Geometry: final body of the model. Coordinates: model frame, mm. Face numbers are marked on the shaded views. A direction names the side the tool comes from. Round coordinates to 2 decimals unless told otherwise and drop trailing zeros. Loops run counter-clockwise (first coordinate to the right, second up) from the corner with the lowest first, then second, coordinate; pieces in that order, holes last. Notation, with made-up numbers: (-17.5, 50.25) - (-0.5, 50.25) arc R38 cw to (-0.5, 88.25) - close; hole circle Ø6 at (25.5, -12). An arc over 180 degrees is marked (long way). Use CSV: the item, a comma, the result in double quotes.
from build123d import *

# Parameters (mm, degrees)
F1_DEPTH  = 60
F2_R      = 22.25
F3_DEPTH  = 4
F4_R      = 4.25
F5_DEPTH  = 25
F6_R      = 8
F7_DEPTH  = 1
F8_SIZE   = 3.74999
F9_R      = 4.25
F10_DEPTH = 25
F11_R     = 8
F12_DEPTH = 1
F13_SIZE  = 3.74999
F14_R     = 5
F15_R     = 7


# Not quite as in the source:
# - a fillet or chamfer is up to 0.001 mm smaller than in the source, because OpenCascade refuses the exact size


with BuildPart() as f1:
    # F0 (on Right) → F1 (new body)
    with BuildSketch(Plane.YZ):
        Polygon((32.3616418088, -17.0859274204), (32.3616418088, 47.9140725796), (22.3616418088, 47.9140725796), (22.3616418088, -7.0859274204), (-22.6383581912, -7.0859274204), (-22.6383581912, -17.0859274204), align=None)
    extrude(amount=F1_DEPTH)

    # F2 (on face) → F3 (join)
    with BuildSketch(Plane(origin=(0, 0, -17.0859274204), x_dir=(1, 0, 0), z_dir=(0, 0, -1))):
        with Locations((30, -4.8616418088)):
            Circle(F2_R)
    extrude(amount=F3_DEPTH)

    # F4 (on face) → F5 (cut)
    with BuildSketch(Plane(origin=(0, 0, -21.0859274204), x_dir=(1, 0, 0), z_dir=(0, 0, -1))):
        with Locations((30, -4.8616418088)):
            Circle(F4_R)
    extrude(amount=-F5_DEPTH, mode=Mode.SUBTRACT)

    # F6 (on face) → F7 (cut)
    with BuildSketch(Plane.XY.offset(-7.0859274204)):
        with Locations((30, 4.8616418088)):
            Circle(F6_R)
    extrude(amount=-F7_DEPTH, mode=Mode.SUBTRACT)

    # F8 (size 3.75 in the source; OpenCascade refuses exactly that, so slightly less here)
    f8_edges = [f1.edges().sort_by_distance(p)[0] for p in [
        (25.75, 4.861642, -8.085927),
    ]]
    chamfer(f8_edges, length=F8_SIZE)

    # F9 (on face) → F10 (cut)
    with BuildSketch(Plane(origin=(0, 32.3616418088, 0), x_dir=(-1, 0, 0), z_dir=(0, 1, 0))):
        with Locations((-30, 25.9140725796)):
            Circle(F9_R)
    extrude(amount=-F10_DEPTH, mode=Mode.SUBTRACT)

    # F11 (on face) → F12 (cut)
    with BuildSketch(Plane(origin=(0, 32.3616418088, 0), x_dir=(-1, 0, 0), z_dir=(0, 1, 0))):
        with Locations((-30, 25.9140725796)):
            Circle(F11_R)
    extrude(amount=-F12_DEPTH, mode=Mode.SUBTRACT)

    # F13 (size 3.75 in the source; OpenCascade refuses exactly that, so slightly less here)
    f13_edges = [f1.edges().sort_by_distance(p)[0] for p in [
        (34.25, 31.361642, 25.914073),
    ]]
    chamfer(f13_edges, length=F13_SIZE)

    # F14
    f14_edges = [f1.edges().sort_by_distance(p)[0] for p in [
        (0, -22.638358, -12.085927),
        (60, -22.638358, -12.085927),
        (60, 27.361642, 47.914073),
        (0, 27.361642, 47.914073),
    ]]
    fillet(f14_edges, radius=F14_R)

    # F15
    f15_edges = [f1.edges().sort_by_distance(p)[0] for p in [
        (30, 22.361642, -7.085927),
    ]]
    fillet(f15_edges, radius=F15_R)


solid = f1.part
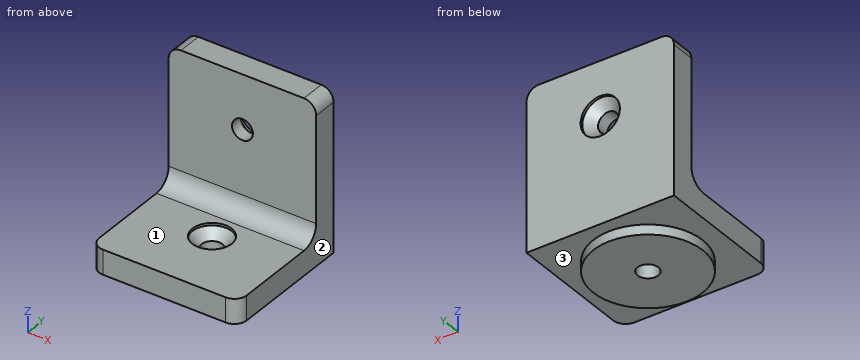
Item 1: Material intervals for line 1 (Z direction, x = 30, y = 32); line 2 (Z direction, x = 30, y = 26.6); line 3 (Y direction, x = 30, z = -18), sorted ascending.
Final values:
line 1,"z = -17.09 to 17.91, 33.91 to 47.91"
line 2,"z = -21.09 to 21.66, 30.16 to 47.91"
line 3,"y = -17.39 to 0.61, 9.11 to 27.11"
Item 2: Section D-D on x = 19.5. Return the cut outline in (y, z) (3 decimals), plus the area to 3 significant figures.
Final values:
outline,"(-22.638, -17.086) - (-14.755, -17.086) - (-14.755, -21.086) - (24.478, -21.086) - (24.478, -17.086) - (32.362, -17.086) - (32.362, 47.914) - (22.362, 47.914) - (22.362, -0.086) arc R7 cw to (15.362, -7.086) - (-22.638, -7.086) - close"
area,"1,270 mm²"
Item 3: Section C-C on z = -13. Return the cut outline in (x, y), plus the area to 3 significant figures.
Final values:
outline,"(0, -17.64) arc R5 ccw to (5, -22.64) - (55, -22.64) arc R5 ccw to (60, -17.64) - (60, 32.36) - (0, 32.36) - close; hole circle Ø8.5 at (30, 4.86)"
area,"3,230 mm²"
Item 4: Pin query (flat end, axial travel): P1, Ø5, axis at x = 30, y = 4.86, coming from the +Z side; P2, Ø10, axis at x = 33, z = 14, coming from the -Y side; P3, Ø8, axis at x = 31, y = 5.5, coming from the +Z side; P4, Ø19, axis at x = 38, y = 2, coming from the +Z side. Return the tip coordinate at first contact, or that it passes through.
Final values:
P1,"passes through"
P2,"stops at y = 22.36"
P3,"stops at z = -10.9"
P4,"stops at z = -7.09"
Item 5: Section B-B on y = -5.5. Return the cut outline in (x, z), plus the area to 3 significant figures.
Final values:
outline,"(0, -17.09) - (10.31, -17.09) - (10.31, -21.09) - (49.69, -21.09) - (49.69, -17.09) - (60, -17.09) - (60, -7.09) - (0, -7.09) - close"
area,"758 mm²"
Item 6: Section A-A on x = 30. Give the number of separate pieces and of enclosed holes in the cut face, plus the area to 3 significant figures.
Final values:
separate pieces,"3"
enclosed holes,"0"
area,"1,040 mm²"
Item 7: Reachability of the marked faces 1, 2 and 3 from +Z, -Z, +X, -X, +Y, -Y: full face, straight path, thin tool, end or side. Return the list, or none.
Final values:
face 1,"+Z, +X, -X, -Y"
face 2,"+Z, -Z, +X, +Y, -Y"
face 3,"-Z"
